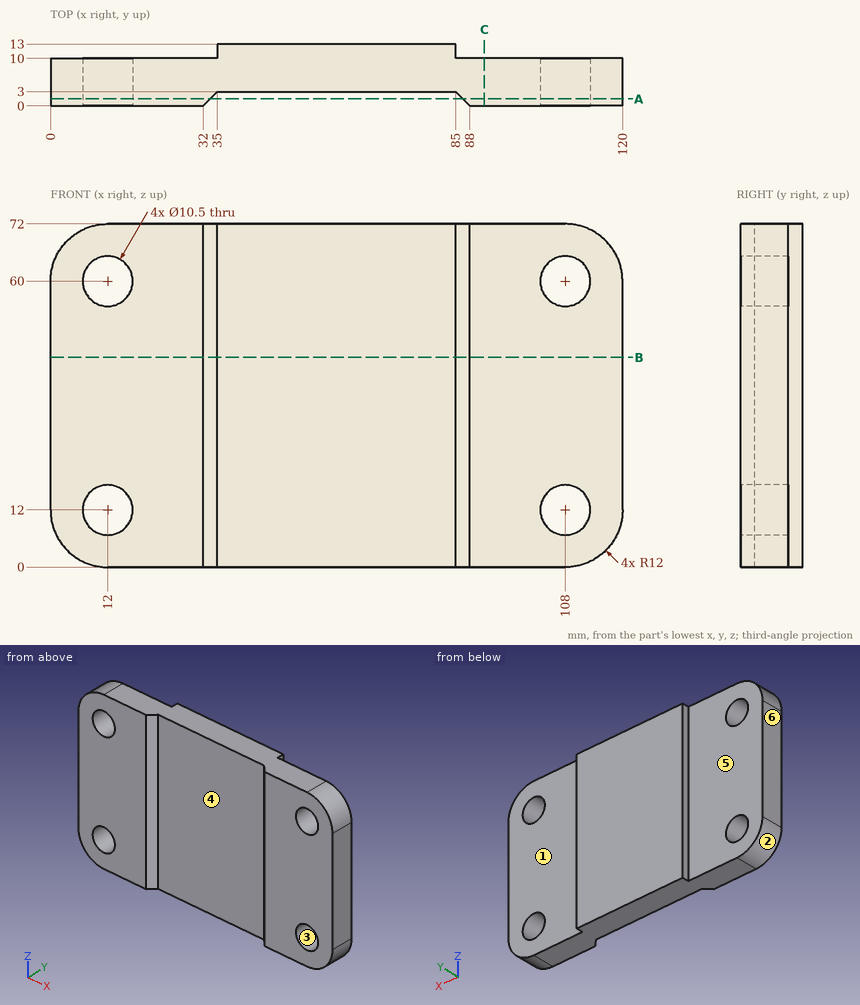
Answer from the drawing. Dimensions are ordinates in mm from the lowest x, y and z of the part. A direction names the side the tool comes from. Round coordinates to 2 decimals unless told otherwise and drop trailing zeros. Loops run counter-clockwise (first coordinate to the right, second up) from the corner with the lowest first, then second, coordinate; pieces in that order, holes last. Notation, with made-up numbers: M 8,68 L 12,68 A24 ccw 12,95 Z; hole C -38,47 d5. An arc over 180 degrees is marked long. One line per question, with ' | ' between items. Start each with the question number.
(1) Find the intervals of material crossed by line 1 (Z direction, x = 108.5, y = 9.5); line 2 (X direction, y = 3.5, z = 12); line 3 (Z direction, x = 111.5, y = 8), in increasing order.
(2) A tool of negligible diameter and unlimited length cuts with its end or side. For the marked faces 5 and 6, from which of +Z, -Z, +X, -X, +Y, -Y can it reach the whole face along a straight path? Write none if from no direction.
(3) For a pull along X with two mould halves and no side action, classify the marked faces 1, 2, 3 and 4 as released by +X, released by -X, zero draft, split by the parting line, or undercut.
(4) A cutting plane is placed at A-A on y = 1.5. Write down the section's boundary in (x, z).
(5) A cutting plane is placed at B-B on z = 44. Write down the section's boundary in (x, y), plus the area to 3 significant figures.
(6) A cutting plane is placed at C-C on x = 91. Write down the section's boundary in (y, z).
(7) Flat-ended cylindrical pins translate along their axes: pin 1 Ø10.5 at (x, z) = (104, 54) entering from +Y; pin 2 Ø1.5 at (y, z) = (11, 21.5) entering from +X; pin 3 Ø3 at (x, z) = (89.5, 14.5) entering from -Y. Find the tip coordinate at first contact, or state that the pin passes through.
Geometry check:
1) line 1: z = 0.01 to 6.77, 17.23 to 54.77, 65.23 to 71.99 | line 2: x = 0 to 6.75, 17.25 to 102.75, 113.25 to 120 | line 3: z = 0.52 to 8.09, 15.91 to 56.09, 63.91 to 71.48
2) face 5: +Z, -Z, -X, +Y | face 6: +Z, -Z, -X, +Y, -Y
3) face 1: zero draft | face 2: released by -X | face 3: undercut | face 4: undercut
4) outline: M 0,12 A12 ccw 12,0 L 33.5,0 L 33.5,72 L 12,72 A12 ccw 0,60 Z; M 86.5,0 L 108,0 A12 ccw 120,12 L 120,60 A12 ccw 108,72 L 86.5,72 Z; hole C 12,12 d10.5; hole C 12,60 d10.5; hole C 108,12 d10.5; hole C 108,60 d10.5
5) outline: M 0,0 L 32,0 L 35,3 L 85,3 L 88,0 L 120,0 L 120,10 L 85,10 L 85,13 L 35,13 L 35,10 L 0,10 Z | area: 1,190 mm²
6) outline: M 0,0 L 10,0 L 10,72 L 0,72 Z
7) pin 1: stops at y = 10 | pin 2: stops at x = 85 | pin 3: stops at y = 0
